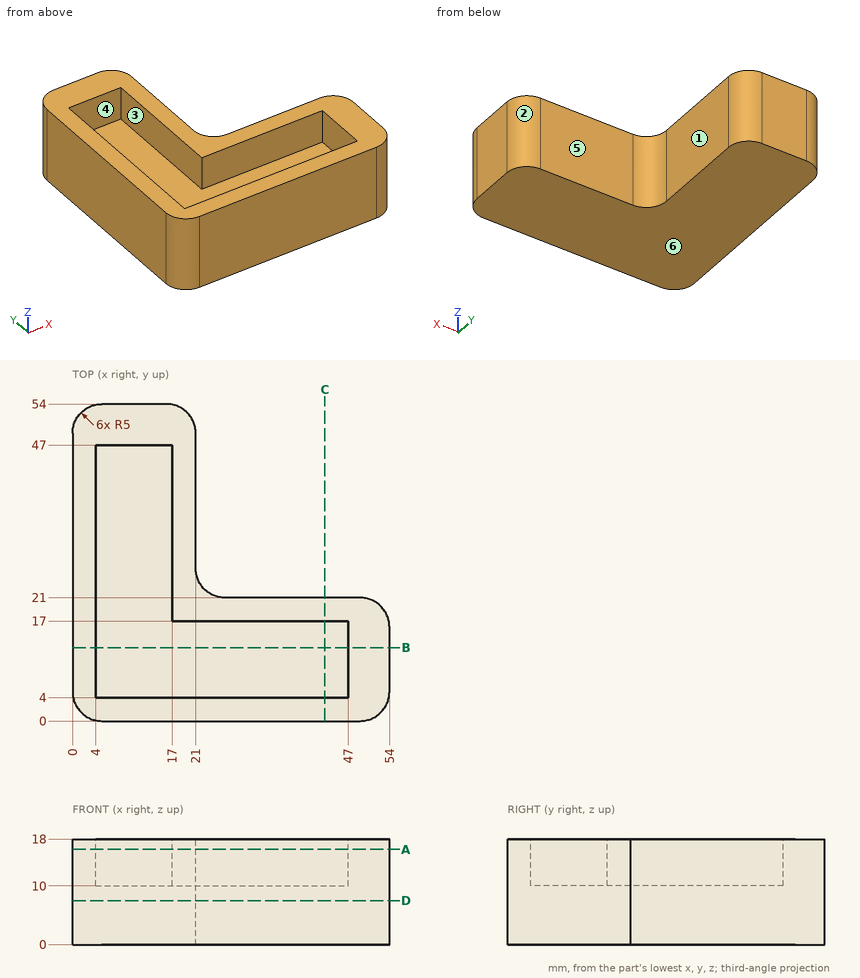
Verification items for this drawing (mm, ordinates from the low corner). A direction names the side the tool comes from. Round coordinates to 2 decimals unless told otherwise and drop trailing zeros. Order: outer loops, then holes, each group sorted by start corner. A loop starts at its lowest first (then second) coordinate and runs counter-clockwise, first axis right, second up. Notation, with made-up numbers: (-20, -27) - (30, -27) arc R25 cw to (30, 10) - close; hole circle Ø10 at (-15, 39.25). An arc over 180 degrees is marked (long way). Answer as CSV lines item,"result". Start each with the question number.
1) Section check B-B (y = 12.5). Record the cut outline in (x, z), then the cut area to 3 significant figures.
2) Section check C-C (x = 43). Record the cut outline in (y, z), then the cut area to 3 significant figures.
3) Section check A-A (z = 16.25). Record the cut outline in (x, y).
4) Section check D-D (z = 7.5). Record the cut outline in (x, y).
5) Draft check along Y on the marked faces 1, 2 and 3. Enter one of: +Y half, -Y half, draft (parallel to the pull), parting line (faces both ways), or undercut.
6) Scan lines: probe 1 along X at (y, z) = (31.5, 16.5); probe 2 along Y at (x, z) = (37, 8); probe 3 along Z at (x, y) = (29, 14). Record each from-to range of solid material in increasing order.
7) Tool access check on the marked faces 4, 5 and 6. Record the directions out of +Z, -Z, +X, -X, +Y, -Y that give a thin tool (end or side, any length) a straight path to the whole face; none if there is none.
8) Depth check by flat-ended pin: pin 1 (6 mm diameter, centred on x = 30, z = 8.5, fed in from +Y); pin 2 (8 mm diameter, centred on x = 9.5, y = 25, fed in from +Z); pin 3 (6.5 mm diameter, centred on y = 32.5, z = 14.5, fed in from +X). Enter the tip coordinate at first touch or a pass-through.
Determined:
1,outline,"(0, 0) - (54, 0) - (54, 18) - (47, 18) - (47, 10) - (4, 10) - (4, 18) - (0, 18) - close"
1,area,"628 mm^2"
2,outline,"(0, 0) - (21, 0) - (21, 18) - (17, 18) - (17, 10) - (4, 10) - (4, 18) - (0, 18) - close"
2,area,"274 mm^2"
3,outline,"(0, 5) arc R5 ccw to (5, 0) - (49, 0) arc R5 ccw to (54, 5) - (54, 16) arc R5 ccw to (49, 21) - (26, 21) arc R5 cw to (21, 26) - (21, 49) arc R5 ccw to (16, 54) - (5, 54) arc R5 ccw to (0, 49) - close; hole (4, 4) - (47, 4) - (47, 17) - (17, 17) - (17, 47) - (4, 47) - close"
4,outline,"(0, 5) arc R5 ccw to (5, 0) - (49, 0) arc R5 ccw to (54, 5) - (54, 16) arc R5 ccw to (49, 21) - (26, 21) arc R5 cw to (21, 26) - (21, 49) arc R5 ccw to (16, 54) - (5, 54) arc R5 ccw to (0, 49) - close"
5,face 1,"draft"
5,face 2,"+Y half"
5,face 3,"undercut"
6,probe 1,"0 to 4, 17 to 21"
6,probe 2,"0 to 21"
6,probe 3,"0 to 10"
7,face 4,"+Z"
7,face 5,"+Z, -Z, +X, +Y"
7,face 6,"-Z, +X, -X, +Y, -Y"
8,pin 1,"y = 21"
8,pin 2,"z = 10"
8,pin 3,"x = 21"
